For this review, take the finished solid that the model builds, in its own axes (mm). Face numbers are marked on the shaded views. A direction names the side the tool comes from. Round coordinates to 2 decimals unless told otherwise and drop trailing zeros. Write each loop counter-clockwise with the first axis right and the second up, starting at its lowest first coordinate (ties: lowest second). Pieces come first, ordered by that corner, then holes. Notation, with made-up numbers: (-32.75, -10.75) -> (-14.75, -10.75) arc R8 ccw to (-14.75, -5.75) -> close; hole circle Ø9 at (-22, 13). An arc over 180 degrees is marked (long way). Write each question's results on one line, items separated by ' | '. Start each with the question number.
Item 1: To check wall thickness, follow line 1 along X through (y, z) = (29, 7.75) (3 decimals); line 2 along Y through (x, z) = (8.5, 3.25); line 3 along Y through (x, z) = (-6, 1.5). State the ranges of each line that lie inside material, in increasing order.
Item 2: Add section A-A (y = 25). State the section outline as (x, z) points (3 decimals), plus the area to 3 significant figures.
Item 3: Clearance check with flat-ended pins moving along their axes: pin 1 (4.5 mm diameter, centred on x = -16, z = 10, fed in from +Y); pin 2 (4 mm diameter, centred on x = 0, y = 18, fed in from -Z); pin 3 (1.5 mm diameter, centred on y = 32, z = 2, fed in from -X). State where each tip first meets the part, or that it passes through.
Item 4: The part is to be moulded in two halves that separate along Y. For the marked faces 1, 2, 3 and 4, say which applies: +Y half, -Y half, draft (parallel to the pull), parting line (faces both ways), or undercut.
Item 5: Add section C-C (x = 4.5). State the section outline as (y, z) points.
Item 6: Add section B-B (x = -1). State the section outline as (y, z) points, plus the area to 3 significant figures.
Item 7: Add section D-D (y = 18). State the section outline as (x, z) points (1 decimal).
Item 8: Tool access review of the marked faces 5, 6, 7, 8 and 9: name each direction out of +Z, -Z, +X, -X, +Y, -Y from which nothing blocks a thin tool from reaching the whole face with its end or side.
Autodesk Inventor part; units mm, degrees
ref_plane "Work Plane4" through (-22.225, 7.62, 15.24) normal (0, 1, 0) x (1, 0, 0)
ref_plane "Work Plane1" through (0, 22.48, 0) normal (-1, 0, 0) x (0, 0, 1)
ref_plane "Work Plane2" through (0, 0, -9.525) normal (0, 0, 1) x (1, 0, 0)
sketch "Sketch1" plane through (0, 0, 0) normal (0, 0, 1) x (1, 0, 0)
  line L0 (0, 57.912) -> (0, -9.652)
  line L1 (-63.881, 0) -> (36.576, 0)
  line L2 (22.225, 48.26) -> (-27.94, 48.26)
  line L3 (-27.94, 48.26) -> (-27.94, 0)
  line L4 (-27.94, 0) -> (22.225, 0)
  line L5 (22.225, 0) -> (22.225, 48.26)
  line L6 (0, 48.26) -> (0, 0) construction
  line L7 (12.7, 48.26) -> (12.7, 0) construction
  line L8 (3.429, 19.305) -> (-3.429, 19.305)
  line L9 (-3.429, 19.305) -> (-3.429, 41.655)
  line L10 (-3.429, 41.655) -> (3.429, 41.655)
  line L11 (3.429, 41.655) -> (3.429, 19.305)
  line L12 (3.429, 19.305) -> (-3.429, 41.655) construction
  line L13 (-3.429, 19.305) -> (3.429, 41.655) construction
  line L14 (16.129, 19.305) -> (9.271, 19.305)
  line L15 (9.271, 19.305) -> (9.271, 41.655)
  line L16 (9.271, 41.655) -> (16.129, 41.655)
  line L17 (16.129, 41.655) -> (16.129, 19.305)
  line L18 (16.129, 19.305) -> (9.271, 41.655) construction
  line L19 (9.271, 19.305) -> (16.129, 41.655) construction
  circle A0 centre (0, 38.48) radius 3.175 construction
  circle A1 centre (0, 30.48) radius 3.175 construction
  line L20 (-27.94, 0) -> (-49.53, 0)
  line L21 (-49.53, 0) -> (-49.53, 7.62)
  line L22 (-49.53, 7.62) -> (-27.94, 7.62)
  line L23 (-27.94, 7.62) -> (-27.94, 0)
  line L24 (-3.9178, 6.35) -> (-23.2802, 6.35)
  line L25 (-23.2802, 6.35) -> (-23.2802, 13.335)
  line L26 (-23.2802, 13.335) -> (-3.9178, 13.335)
  line L27 (-3.9178, 13.335) -> (-3.9178, 6.35)
  line L28 (-3.9178, 6.35) -> (-23.2802, 13.335) construction
  line L29 (-23.2802, 6.35) -> (-3.9178, 13.335) construction
  line L30 (-23.2802, 13.335) -> (-17.0915, 20.955)
  line L31 (-17.0915, 20.955) -> (-10.1065, 20.955)
  line L32 (-10.1065, 20.955) -> (-3.9178, 13.335)
  line L33 (-13.599, 9.8425) -> (-13.599, 20.955) construction
  circle A2 centre (0, 22.48) radius 6.35 construction
  point P0 (0, 0)
  point P1 (0, 25.4)
  point P2 (0, 30.48)
  point P3 (12.7, 30.48)
  point P4 (12.7, 30.48)
  dimension "d0" = 48.26
  dimension "d2" = 6.858
  dimension "d3" = 0
  dimension "d5" = 6.35
  dimension "d6" = 8
  dimension "d27" = 12.7
  dimension "d56" = 41.655
  dimension "d57" = 6.605
  dimension "d58" = 30.48
  dimension "d59" = 7.62
  dimension "d60" = 21.59
  dimension "d61" = 6.985
  dimension "d62" = 6.35
  dimension "d64" = 13.599
  dimension "d81" = 22.225
  dimension "d82" = 27.94
  dimension "d84" = 6.985
  dimension "d85" = 3.4925
  dimension "d86" = 7.62
  dimension "d104" = 12.7
  dimension "d105" = 8
  dimension "d119" = 13.599
extrude "Extrusion1" add sketch "Sketch1" along normal blind 15.24 contours L2 L5 L1 L0 L8 L11 L10 | L0 L10 L9 L8 L1 L3 L2 | L24 L25 L26 L27 | L26 L30 L31 L32
ref_plane "Work Plane4" through (-22.225, 7.62, 15.24) normal (0, 1, 0) x (1, 0, 0)
sketch "Sketch4" plane through (-22.225, 7.62, 15.24) normal (0, 1, 0) x (1, 0, 0)
  line L0 (-23.495, 8.255) -> (0, 8.255)
  line L1 (-23.495, 8.255) -> (-23.495, -17.78)
  line L2 (-23.495, 8.255) -> (-14.605, 8.255)
  line L3 (-14.605, 8.255) -> (-14.605, 0)
  line L4 (-14.605, 0) -> (-23.495, 0)
  line L5 (-23.495, 0) -> (-23.495, 8.255)
  line L6 (44.45, 0) -> (0, 0)
  point P0 (22.225, 15.24)
  dimension "d28" = 0
  dimension "d29" = 8.89
extrude "Extrusion4" [suppressed]
fillet "Fillet1" radius 3.175 8 edges at (-3.429, 19.305, 7.62) (3.429, 19.305, 7.62) (3.429, 41.655, 7.62) (-3.429, 41.655, 7.62) (9.271, 41.655, 7.62) (16.129, 41.655, 7.62) (16.129, 19.305, 7.62) (9.271, 19.305, 7.62)
ref_plane "Work Plane1" through (0, 22.48, 0) normal (-1, 0, 0) x (0, 0, 1)
ref_plane "Work Plane2" through (0, 0, -9.525) normal (0, 0, 1) x (1, 0, 0)
extrude "Extrusion8" cut sketch "Sketch1" along normal up to next contours L24 L25 L26 L27 | L26 L30 L31 L32
ref_plane "Work Plane5" through (-13.599, 6.35, 15.24) normal (1, 0, 0) x (0, 0, -1)
sketch "Sketch7" plane through (22.225, 0, 0) normal (0, -1, 0) x (1, 0, 0)
  line L0 (0, 0) -> (0, 15.24)
  line L1 (-50.165, 15.24) -> (0, 15.24)
  line L2 (-50.165, 0) -> (0, 0)
  line L3 (-71.755, 7.62) -> (0, 7.62) construction
  line L4 (-53.204, 3.81) -> (-68.444, 3.81)
  line L5 (-68.444, 3.81) -> (-68.444, 11.43)
  line L6 (-68.444, 11.43) -> (-53.204, 11.43)
  line L7 (-53.204, 11.43) -> (-53.204, 3.81)
  line L8 (-53.204, 3.81) -> (-68.444, 11.43) construction
  line L9 (-68.444, 3.81) -> (-53.204, 11.43) construction
  line L10 (-43.444, 3.81) -> (-28.204, 3.81)
  line L11 (-28.204, 3.81) -> (-28.204, 11.43)
  line L12 (-28.204, 11.43) -> (-43.444, 11.43)
  line L13 (-43.444, 11.43) -> (-43.444, 3.81)
  line L14 (-43.444, 3.81) -> (-28.204, 11.43) construction
  line L15 (-28.204, 3.81) -> (-43.444, 11.43) construction
  line L16 (-50.165, 0) -> (0, 0)
  line L17 (0, 0) -> (0, 15.24)
  line L18 (-50.165, 15.24) -> (0, 15.24)
  line L19 (-45.5052, 0) -> (-26.1428, 0)
  line L20 (-26.1428, 15.24) -> (-45.5052, 15.24)
  line L21 (-45.5052, 0) -> (-45.5052, 15.24)
  line L22 (-26.1428, 0) -> (-26.1428, 15.24)
  line L23 (-35.824, 18.288) -> (-35.824, -3.048)
  line L24 (-50.165, 0) -> (-50.165, 15.24)
  line L25 (-22.225, 18.288) -> (-22.225, -3.048)
  point P0 (-22.225, 0)
  point P1 (-60.824, 7.62)
  point P2 (-35.824, 7.62)
  point P3 (-22.225, 0)
  point P4 (-22.225, 0)
  point P5 (-22.225, 0)
  point P6 (-25.856, 0)
  point P7 (-35.824, 7.62)
  dimension "d69" = 7.62
  dimension "d70" = 15.24
  dimension "d71" = 25
  dimension "d88" = 0
  dimension "d120" = 9.6812
extrude "Extrusion10" cut sketch "Sketch7" against normal up to surface (6.35 mm away) contours L23 L12 L11 L10 | L10 L13 L12 L23
sketch "Sketch9" plane through (0, 0, 0) normal (0, 0, 1) x (1, 0, 0)
  line L0 (-10.1063, 6.35) -> (-27.94, 6.35)
  line L1 (-27.94, 6.35) -> (-27.94, 48.26)
  line L2 (-27.94, 48.26) -> (-10.1063, 48.26)
  line L3 (-10.1063, 48.26) -> (-10.1063, 6.35)
  line L4 (-3.9178, 6.35) -> (-23.2802, 6.35)
  point P0 (0, 0)
  dimension "d101" = 0
extrude "Extrusion12" cut sketch "Sketch9" along normal up to next
fillet "Fillet15" radius 3.175 4 edges at (-5.979, 3.175, 3.81) (-5.979, 3.175, 11.43) (-21.219, 3.175, 11.43) (-21.219, 3.175, 3.81)
sketch "Sketch10" plane through (0, 0, 0) normal (0, 0, -1) x (-1, 0, 0)
  line L0 (10.1065, 20.955) -> (3.9178, 13.335)
  line L1 (3.9178, 6.35) -> (3.9178, 13.335)
  line L2 (27.94, 6.35) -> (3.9178, 6.35)
  line L3 (10.1065, 20.955) -> (10.1065, 6.35)
  line L4 (3.9178, 6.35) -> (27.94, 6.35)
  point P0 (0, 0)
extrude "Extrusion13" add sketch "Sketch10" against normal blind 1.016
sketch "Sketch11" plane through (0, 0, 15.24) normal (0, 0, 1) x (1, 0, 0)
  line L0 (-10.1065, 20.955) -> (-10.1065, 6.35)
  line L1 (-10.1063, 20.9547) -> (-3.9178, 13.335)
  line L2 (-3.9178, 13.335) -> (-3.9178, 6.35)
  line L3 (-3.9178, 6.35) -> (-27.94, 6.35)
  line L4 (-10.1063, 20.9547) -> (-10.1065, 6.35)
  point P0 (0, 0)
extrude "Extrusion14" add sketch "Sketch11" against normal blind 1.016
fillet "Fillet18" radius 3.175 2 edges at (-3.9178, 9.8425, 1.016) (-3.9178, 9.8425, 14.224)
fillet "Fillet19" radius 3.175 2 edges at (-27.94, 3.175, 0) (-27.94, 3.175, 15.24)
fillet "Fillet20" radius 3.175 2 edges at (-10.1065, 6.35, 14.732) (-10.1065, 6.35, 0.508)
sketch "Sketch12" plane through (0, 0, 0) normal (0, 0, -1) x (-1, 0, 0)
  line L0 (-12.7, 30.48) -> (0, 30.48) construction
  line L1 (0.254, 15.876) -> (-12.954, 15.876)
  line L2 (-19.304, 22.226) -> (-19.304, 38.734)
  line L3 (-12.954, 45.084) -> (0.254, 45.084)
  line L4 (6.604, 38.734) -> (6.604, 22.226)
  line L5 (6.604, 15.876) -> (-19.304, 45.084) construction
  line L6 (-19.304, 15.876) -> (6.604, 45.084) construction
  arc A0 (-12.954, 45.084) -> (-19.304, 38.734) centre (-12.954, 38.734) ccw
  arc A1 (6.604, 38.734) -> (0.254, 45.084) centre (0.254, 38.734) ccw
  arc A2 (0.254, 15.876) -> (6.604, 22.226) centre (0.254, 22.226) ccw
  arc A3 (-19.304, 22.226) -> (-12.954, 15.876) centre (-12.954, 22.226) ccw
  point P0 (0, 0)
  point P1 (-6.35, 30.48)
  dimension "d113" = 6.604
  dimension "d114" = 14.604
  dimension "d115" = 6.35
extrude "Extrusion15" cut sketch "Sketch12" against normal blind 5.08
fillet "Fillet21" radius 6.35 2 edges at (22.225, 48.26, 7.62) (-10.1063, 48.26, 7.62)
equation "\"d85\" = 0.5 * d84"
properties part number "J005556" material "VERO BLACK"
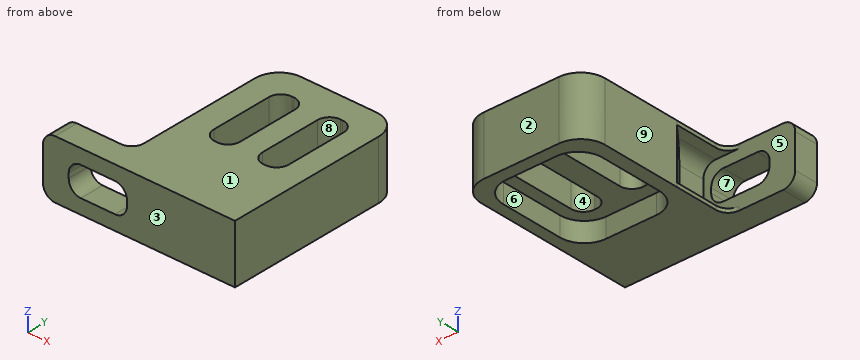
Responses:
1) line 1: x = -10.106 to -3.429, 3.429 to 9.271, 16.129 to 22.225 | line 2: y = 0 to 15.88, 45.08 to 48.26 | line 3: y = 0 to 6.35, 15.9 to 19.52, 41.44 to 47.85
2) outline: (-10.106, 0) -> (-6.604, 0) -> (-6.604, 5.08) -> (-3.429, 5.08) -> (-3.429, 15.24) -> (-10.106, 15.24) -> close; (3.429, 5.08) -> (9.271, 5.08) -> (9.271, 15.24) -> (3.429, 15.24) -> close; (16.129, 5.08) -> (19.304, 5.08) -> (19.304, 0) -> (22.225, 0) -> (22.225, 15.24) -> (16.129, 15.24) -> close | area: 222 mm^2
3) pin 1: stops at y = 6.35 | pin 2: stops at z = 5.08 | pin 3: stops at x = -10.11
4) face 1: draft | face 2: +Y half | face 3: -Y half | face 4: undercut
5) outline: (0, 0) -> (15.88, 0) -> (15.88, 5.08) -> (45.08, 5.08) -> (45.08, 0) -> (48.26, 0) -> (48.26, 15.24) -> (0, 15.24) -> close
6) outline: (0, 0) -> (15.92, 0) -> (15.92, 5.08) -> (19.39, 5.08) -> (19.39, 15.24) -> (0, 15.24) -> close; (41.57, 5.08) -> (45.04, 5.08) -> (45.04, 0) -> (48.26, 0) -> (48.26, 15.24) -> (41.57, 15.24) -> close | area: 362 mm^2
7) outline: (-10.1, 0) -> (-5, 0) -> (-5, 5.1) -> (17.7, 5.1) -> (17.7, 0) -> (22.2, 0) -> (22.2, 15.2) -> (-10.1, 15.2) -> (-10.1, 14.2) -> (-7.7, 14.2) -> (-7.7, 1) -> (-10.1, 1) -> close
8) face 5: -X | face 6: -Z | face 7: -Y | face 8: +Z, -Z | face 9: +Z, -Z, -X, +Y
